Study the drawing (mm; zero at the part's minimum x, y, z) and answer. A direction names the side the tool comes from. Give positions to 0.01 mm unless a question says otherwise; leave off trailing zeros. Order: outer loops, then holes, each group sorted by start corner. A loop starts at its lowest first (then second) coordinate and runs counter-clockwise, first axis right, second up. Notation, with made-up numbers: (7, 79) - (17, 79) arc R20 ccw to (17, 95) - close; hole circle Ø5 at (-29.75, 45). An arc over 180 degrees is marked (long way). Put each result on its own line as item: value.
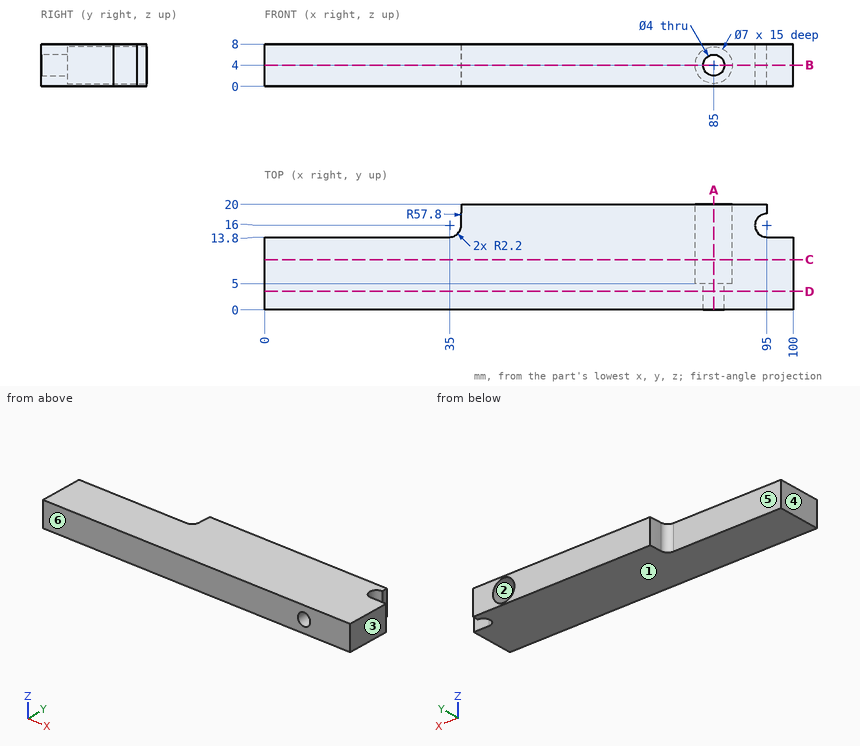
(1) A tool of negligible diameter and unlimited length cuts with its end or side. For the marked faces 5 and 6, from which of +Z, -Z, +X, -X, +Y, -Y can it reach the whole face along a straight path? Write none if from no direction.
Geometry check:
face 5: +Z, -Z, -X, +Y
face 6: +Z, -Z, +X, -X, -Y
(2) Straight lines are drawn through the part: line 1 (X direction, y = 10, z = 4); line 2 (X direction, y = 1.5, z = 4); line 3 (Y direction, x = 12, z = 7.5). For each, find the intervals that lie inside material, in ascending order.
Geometry check:
line 1: x = 0 to 81.5, 88.5 to 100
line 2: x = 0 to 83, 87 to 100
line 3: y = 0 to 13.8
(3) Section B-B, the plane z = 4 is taken. Write down the section's boundary in (x, y), then the cut area to 3 significant figures.
Geometry check:
outline: (0, 0) - (83, 0) - (83, 5) - (81.5, 5) - (81.5, 20) - (37.34, 20) arc R57.8 ccw to (37.2, 16) arc R2.2 cw to (35, 13.8) - (0, 13.8) - close; (87, 0) - (100, 0) - (100, 13.8) - (95, 13.8) arc R2.2 cw to (95, 18.2) - (95, 20) - (88.5, 20) - (88.5, 5) - (87, 5) - close
area: 1,610 mm²
(4) Section D-D, the plane y = 3.5 is taken. Write down the section's boundary in (x, z).
Geometry check:
outline: (0, 0) - (100, 0) - (100, 8) - (0, 8) - close; hole circle Ø4 at (85, 4)
(5) Section C-C, the plane y = 9.5 is taken. Write down the section's boundary in (x, z).
Geometry check:
outline: (0, 0) - (100, 0) - (100, 8) - (0, 8) - close; hole circle Ø7 at (85, 4)
(6) Given pin 1 (4 mm diameter, centred on x = 18.5, z = 5.5, fed in from +Y); pin 2 (5 mm diameter, centred on x = 14, y = 4, fed in from -Z); pin 3 (0.5 mm diameter, centred on y = 19.5, z = 3.5, fed in from +X); pin 4 (4 mm diameter, centred on y = 17.5, z = 1, fed in from -X), each flat-ended and moving along its own axis, determine where each tip first touches the part or whether it passes through.
Geometry check:
pin 1: stops at y = 13.8
pin 2: stops at z = 0
pin 3: stops at x = 95
pin 4: stops at x = 37.14
(7) Determine the mould class of the marked faces 1, 2, 3 and 4 for opening direction X: pulls with the +X half, pulls with the -X half, needs draft (parallel to the pull), parting line crosses it, or undercut.
Geometry check:
face 1: needs draft
face 2: undercut
face 3: pulls with the +X half
face 4: pulls with the -X half
(8) Section A-A, the plane x = 85 is taken. Write down the section's boundary in (y, z).
Geometry check:
outline: (0, 0) - (20, 0) - (20, 0.5) - (5, 0.5) - (5, 2) - (0, 2) - close; (0, 6) - (5, 6) - (5, 7.5) - (20, 7.5) - (20, 8) - (0, 8) - close
